For this review, use the dimensioned drawing (mm, ordinates from the lowest corner) and the shaded views. A direction names the side the tool comes from. Coordinates: 2 decimals unless noted, no trailing zeros. Write each loop counter-clockwise with the first axis right and the second up, starting at its lowest first coordinate (ties: lowest second). Pieces come first, ordered by that corner, then holes. Notation, with made-up numbers: (20.25, 4) - (39.25, 4) arc R24 ccw to (39.25, 14) - close; hole circle Ø6 at (60, -12.75). An arc over 180 degrees is marked (long way). One line per item, written item: value.
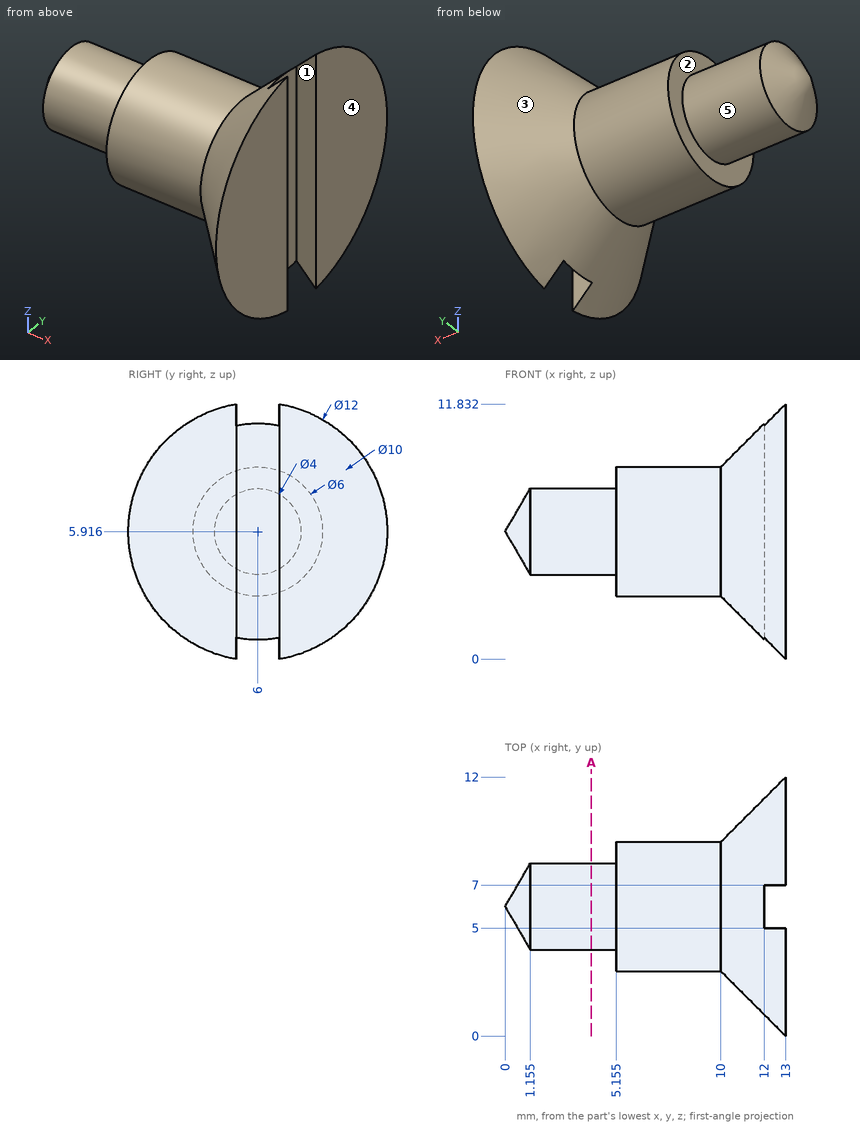
1. Consider section A-A, the plane x = 4. Write out the cut boundary in (y, z).
Answer block:
outline: circle Ø4 at (6, 5.92)
2. For the marked faces 4 and 5, list the 3-axis set-ups (+Z, -Z, +X, -X, +Y, -Y) from which the entire face can be reached by the end or side of a thin tool; tool diameter is ignored.
Answer block:
face 4: +Z, -Z, +X, +Y, -Y
face 5: -X
3. Mouldability with a two-part tool opening along Y and no side actions: class the marked faces 1, 2 and 3 as released by +Y, released by -Y, zero draft, split by the parting line, or undercut.
Answer block:
face 1: undercut
face 2: zero draft
face 3: split by the parting line
4. Insertion check: pin 1 Ø0.5 at (x, z) = (12.5, 7) entering from +Y; pin 2 Ø1.5 at (x, z) = (9.5, 3) entering from +Y (1 decimal); pin 3 Ø4 at (x, y) = (7.5, 8.5) entering from +Z. Each pin has a flat end and moves straight along its axis. Give the tip position at first contact, or say it passes through.
Answer block:
pin 1: stops at y = 11.65
pin 2: stops at y = 8.1
pin 3: stops at z = 8.87
5. Wall thickness on line 1 along X through (y, z) = (6, 3) (1 decimal); line 2 along X through (y, z) = (4, 7.5) (1 decimal); line 3 along Z through (x, y) = (10.75, 4) (1 decimal): over which ranges is each line inside the solid? List them lowest first.
Answer block:
line 1: x = 5.2 to 12
line 2: x = 5.2 to 13
line 3: z = 2.7 to 9.1
